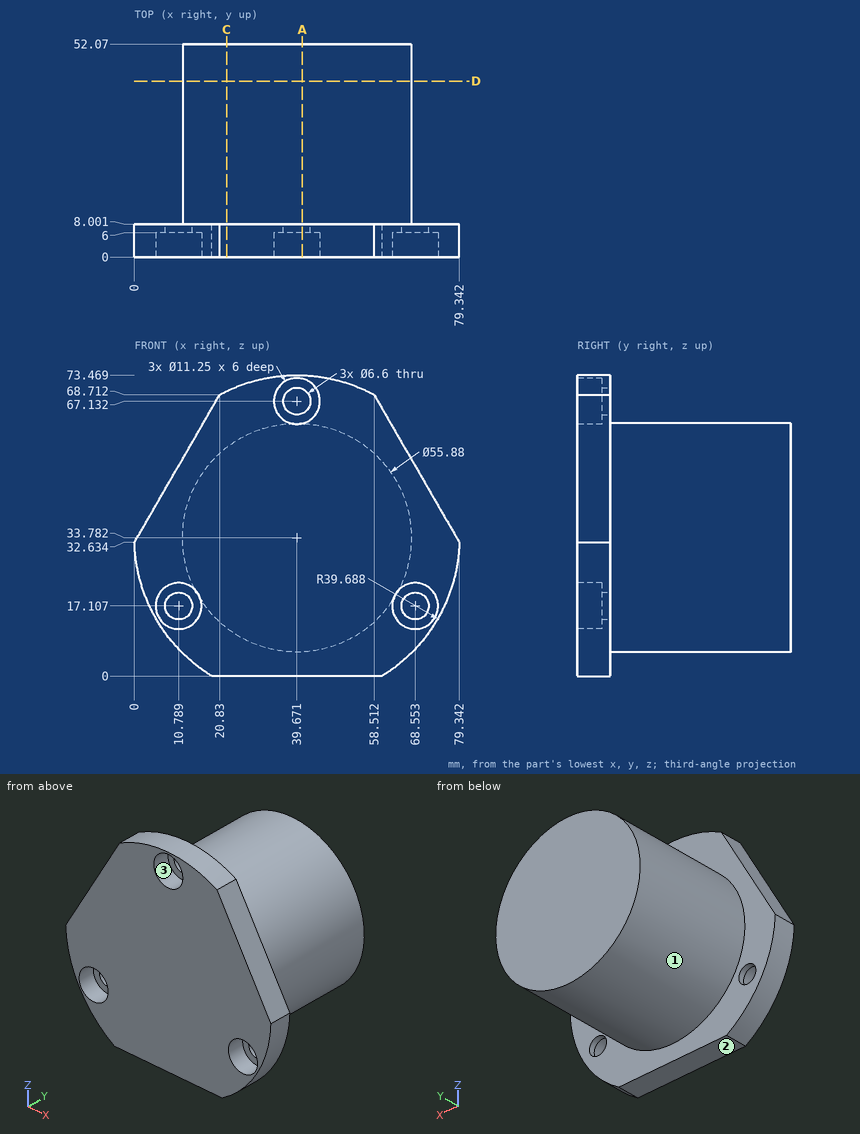
Could you check a few things on this drawing? It's one solid part, dimensions in mm from its lowest x, y, z. A direction names the side the tool comes from. Coordinates: 2 decimals unless noted, no trailing zeros. Order: outer loops, then holes, each group sorted by start corner. A loop starts at its lowest first (then second) coordinate and runs counter-clockwise, first axis right, second up. Notation, with made-up numbers: (-34, 65) - (11, 65) arc R22 cw to (11, 84) - close; hole circle Ø6 at (-1.75, 20). An arc over 180 degrees is marked (long way). Answer as a JSON object with one key per item and string values. Group by question number.
Q1. Imagine slicing it at C-C (x = 22.5). Please give me the cut outline in (y, z).
Q2. Imagine slicing it at D-D (y = 43). Please give me the cut outline in (x, z), and give its area (3 significant figures).
Q3. I need wall thicknesses on line 1 (X direction, y = 35.5, z = 45); line 2 (Y direction, x = 13.5, z = 11); line 3 (Y direction, x = 43.5, z = 70.5). Which ranges of each line are inside material? Lowest first, please. Write a range as from..to.
Q4. Will these pins go through, and if not, where does the flat tip stop? P1, Ø8.5, axis at x = 39.67, z = 67.13, coming from the -Y side; P2, Ø8, axis at x = 48, y = 17.5, coming from the -Z side; P3, Ø1.5, axis at y = 20, z = 63.5, coming from the -X side; P4, Ø6, axis at x = 26, y = 38, coming from the -Z side.
Q5. On a 3-axis mill with a long thin cutter (end or side, diameter ignored), from which of +Z, -Z, +X, -X, +Y, -Y can I reach the whole of each face in a straight line? I mean the marked faces 1, 2 and 3. Say none if no direction works.
Q6. Imagine slicing it at A-A (x = 41). Please give me the cut outline in (y, z), and give its area (3 significant figures).
Determined:
{
 "1": {"outline": "(0, 0) - (8, 0) - (8, 11.74) - (52.07, 11.74) - (52.07, 55.82) - (8, 55.82) - (8, 69.56) - (0, 69.56) - close"},
 "2": {"outline": "circle Ø55.88 at (39.67, 33.78)", "area": "2,450 mm2"},
 "3": {"line 1": "x = 14.08..65.26", "line 2": "y = 0..8", "line 3": "y = 6..8"},
 "4": {"P1": "stops at y = 6", "P2": "stops at z = 6.18", "P3": "passes through", "P4": "stops at z = 7.96"},
 "5": {"face 1": "+Y", "face 2": "-Z, +X, -X, +Y, -Y", "face 3": "-Y"},
 "6": {"outline": "(0, 0) - (8, 0) - (8, 5.87) - (52.07, 5.87) - (52.07, 61.69) - (8, 61.69) - (8, 64.11) - (6, 64.11) - (6, 61.67) - (0, 61.67) - close; (0, 72.6) - (6, 72.6) - (6, 70.15) - (8, 70.15) - (8, 73.45) - (0, 73.45) - close", "area": "2,970 mm2"}
}
